Can you work these out from the model? Positions are in its coordinate system, mm. Face numbers are marked on the shaded views. A direction names the side the tool comes from. Give positions to 0.01 mm unless a question says otherwise; leave off trailing zeros. Order: outer loops, then holes, each group sorted by start corner. A loop starts at its lowest first (then second) coordinate and runs counter-clockwise, first axis right, second up.
Item 1: If we mould it in two halves opening along Y, with no side actions, what happens to the marked faces 6, 7 and 8? For each: +Y half, -Y half, draft (parallel to the pull), parting line (faces both ways), or undercut.
Item 2: I want a section at B-B, the plane y = 1.75. Write out the boundary of the cut face in (x, z).
Item 3: I'm going to push flat-ended pins straight in: pin 1 Ø5 at (x, y) = (0, 0) entering from -Z; pin 2 Ø3.5 at (y, z) = (0, 3.5) entering from +X. Where does each tip first touch, or does it pass through?
Item 4: I want a section at A-A, the plane z = 3.5. Write out the boundary of the cut face in (x, y), then the cut area to 3 significant figures.
Item 5: Which directions (+Z, -Z, +X, -X, +Y, -Y) give clear straight access to the entire face, cutting with the end or side of a thin tool? Please do the marked faces 1, 2, 3, 4 and 5.
Item 6: If I drill on line 1 along X through (y, z) = (3, 3.25); line 2 along Y through (x, z) = (-4.3, 3.5); line 3 along Z through (x, y) = (2.5, 3.25), over which ranges is the centre line in solid material (lowest first)?
Item 7: I want a section at C-C, the plane x = 4.25. Write out the boundary of the cut face in (y, z).
Item 8: I want a section at D-D, the plane y = -3.5. Write out the boundary of the cut face in (x, z).
```python
from build123d import *

# Parameters (mm, degrees)
SKETCH1_W           = 10
SKETCH1_H           = 10
BOSS_EXTRUDE1_DEPTH = 1
SKETCH2_W           = 1
SKETCH2_H           = 10
BOSS_EXTRUDE2_DEPTH = 5
SKETCH3_R           = 2
CUT_EXTRUDE1_DEPTH  = 12
SKETCH4_R           = 5
SKETCH4_R_2         = 4
BOSS_EXTRUDE3_DEPTH = 1


with BuildPart() as part:
    # Sketch1 → Boss-Extrude1 (new body)
    with BuildSketch(Plane.XY):
        Rectangle(SKETCH1_W, SKETCH1_H)
    extrude(amount=BOSS_EXTRUDE1_DEPTH)

    # Sketch2 → Boss-Extrude2 (add)
    with BuildSketch(Plane.XY.offset(1)):
        with Locations((-4.5, 0)):
            Rectangle(SKETCH2_W, SKETCH2_H)
        with Locations((4.5, 0)):
            Rectangle(SKETCH2_W, SKETCH2_H)
    extrude(amount=BOSS_EXTRUDE2_DEPTH)

    # Sketch3 → Cut-Extrude1 (cut)
    with BuildSketch(Plane(origin=(5, 0, 0), x_dir=(0, 0, -1), z_dir=(1, 0, 0))):
        with Locations((-3.5, 0)):
            Circle(SKETCH3_R)
    extrude(amount=-CUT_EXTRUDE1_DEPTH, mode=Mode.SUBTRACT)

    # Sketch4 → Boss-Extrude3 (add)
    with BuildSketch(Plane(origin=(0, 0, 0), x_dir=(-1, 0, 0), z_dir=(0, 0, -1))):
        Circle(SKETCH4_R)
        Circle(SKETCH4_R_2, mode=Mode.SUBTRACT)
    extrude(amount=BOSS_EXTRUDE3_DEPTH)


solid = part.part
```
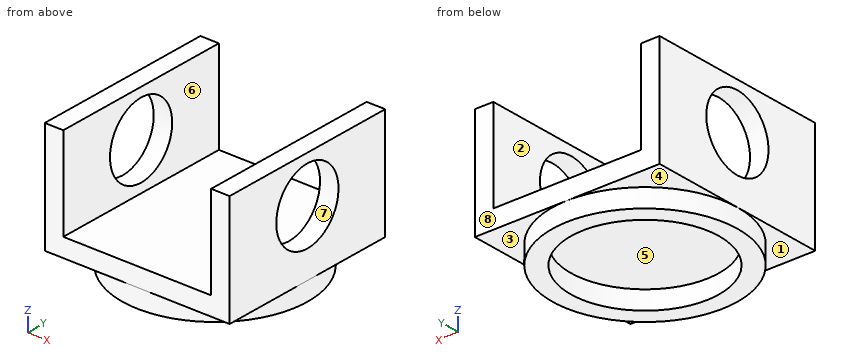
Results list:
1. face 6: draft
1. face 7: undercut
1. face 8: +Y half
2. outline: (-5, 0) - (-4.68, 0) - (-4.68, -1) - (-3.6, -1) - (-3.6, 0) - (3.6, 0) - (3.6, -1) - (4.68, -1) - (4.68, 0) - (5, 0) - (5, 2.53) - (4, 2.53) - (4, 1) - (-4, 1) - (-4, 2.53) - (-5, 2.53) - close; (-5, 4.47) - (-4, 4.47) - (-4, 6) - (-5, 6) - close; (4, 4.47) - (5, 4.47) - (5, 6) - (4, 6) - close
3. pin 1: stops at z = 0
3. pin 2: passes through
4. outline: (-5, -5) - (-4, -5) - (-4, -2) - (-5, -2) - close; (-5, 2) - (-4, 2) - (-4, 5) - (-5, 5) - close; (4, -5) - (5, -5) - (5, -2) - (4, -2) - close; (4, 2) - (5, 2) - (5, 5) - (4, 5) - close
4. area: 12.0 mm2
5. face 1: -Z, -X, -Y
5. face 2: +Z, +Y, -Y
5. face 3: -Z, +X, +Y
5. face 4: -Z, -X, +Y
5. face 5: -Z
6. line 1: x = -5 to -4, 4 to 5
6. line 2: y = -5 to -2, 2 to 5
6. line 3: z = -1 to 1
7. outline: (-5, 0) - (-2.63, 0) - (-2.63, -1) - (2.63, -1) - (2.63, 0) - (5, 0) - (5, 6) - (-5, 6) - close; hole circle Ø4 at (0, 3.5)
8. outline: (-5, 0) - (-3.57, 0) - (-3.57, -1) - (-1.94, -1) - (-1.94, 0) - (1.94, 0) - (1.94, -1) - (3.57, -1) - (3.57, 0) - (5, 0) - (5, 6) - (4, 6) - (4, 1) - (-4, 1) - (-4, 6) - (-5, 6) - close
